Geometry: final body of the model. Coordinates: model frame, mm. Round coordinates to 2 decimals unless told otherwise and drop trailing zeros. Write each question's results on one line, items separated by ' | '.
```python
from build123d import *

# Parameters (mm, degrees)
F7_DEPTH = 50
F8_W     = 5
F8_H     = 5
F9_DEPTH = 12.5


with BuildPart() as f5:
    # F2 (on face) → F5 section 0
    with BuildSketch(Plane(origin=(14.1421356237, 0, 14.1421356237), x_dir=(0.7071067812, 0, -0.7071067812), z_dir=(-0.7071067812, 0, -0.7071067812))):
        Polygon((-9.3261531631, 3.0302508528), (-9.3261531631, -3.0302508528), (-5.7638796391, -7.933299727), (0, -9.8060977485), (5.7638796391, -7.933299727), (9.3261531631, -3.0302508528), (9.3261531631, 3.0302508528), (5.7638796391, 7.933299727), (0, 9.8060977485), (-5.7638796391, 7.933299727), align=None)
    # F4 (on face) → F5 section 1
    with BuildSketch(Plane(origin=(0, 0, 0), x_dir=(0.7071067812, 0, -0.7071067812), z_dir=(-0.7071067812, 0, -0.7071067812))):
        Polygon((-0.0475528258, 0.0154508497), (-0.0475528258, -0.0154508497), (-0.0293892626, -0.0404508497), (0, -0.05), (0.0293892626, -0.0404508497), (0.0475528258, -0.0154508497), (0.0475528258, 0.0154508497), (0.0293892626, 0.0404508497), (0, 0.05), (-0.0293892626, 0.0404508497), align=None)
    loft()

    # F6 (on face) → F7 (join)
    with BuildSketch(Plane(origin=(14.1421356237, 0, 14.1421356237), x_dir=(0.7071067812, 0, -0.7071067812), z_dir=(0.7071067812, 0, 0.7071067812))):
        with BuildLine():
            Line((1.7084597584, -2.4660018763), (1.7084597584, 2.4660018763))
            ThreePointArc((1.7084597584, 2.4660018763), (-3, 0), (1.7084597584, -2.4660018763))
        make_face()
    extrude(amount=F7_DEPTH)

    # F8 (on Front) → F9 (cut, symmetric)
    with BuildSketch(Plane.XZ):
        with Locations((11.3405170292, 22.6421356237)):
            Rectangle(F8_W, F8_H)
    extrude(amount=F9_DEPTH, both=True, mode=Mode.SUBTRACT)


solid = f5.part
```
1. Ray query, probe 1 along X at (y, z) = (-1.25, 20.5); probe 2 along X at (y, z) = (-2, 16); probe 3 along Z at (x, y) = (14.5, 7.25). Return the intervals inside material, ascending.
Answer key:
probe 1: x = 7.46 to 7.78, 16.64 to 22.92 | probe 2: x = 5.81 to 12.28, 12.84 to 18.42 | probe 3: z = 9.62 to 13.78
2. Draft query along X for faces 1 (the face through (49.018, 0.042, 49.977)), 2 (the face through (15.487, 0.755, 12.798)). Return one class per face: pulls with the +X half, pulls with the -X half, needs draft (parallel to the pull), parting line crosses it, or undercut.
Answer key:
face 1: pulls with the +X half | face 2: undercut
3. Pin query (flat end, axial travel): P1, Ø5, axis at y = 6.5, z = 11.5, coming from the -X side; P2, Ø8, axis at x = 5.5, y = -1, coming from the +Z side; P3, Ø5, axis at x = 32, z = 25.5, coming from the -Y side; P4, Ø10, axis at x = 35, z = 37.5, coming from the +Y side. Return the tip coordinate at first contact, or that it passes through.
Answer key:
P1: stops at x = 5.54 | P2: stops at z = 20.74 | P3: passes through | P4: stops at y = 3
